from build123d import *


with BuildPart() as part:
    # Sketch1 → Base-Revolve (revolve)
    with BuildSketch(Plane.XY):
        with BuildLine():
            Line((163, 32.5), (0, 32.5))
            Line((0, 32.5), (-162.6, 32.5))
            ThreePointArc((-162.6, 32.5), (-162.882842712, 32.382842712), (-163, 32.1))
            Line((-163, 32.1), (-163, 28.4))
            ThreePointArc((-163, 28.4), (-163.117157288, 28.117157288), (-163.4, 28))
            Line((-163.4, 28), (-164, 28))
            Line((-164, 28), (-164, 25.230940108))
            ThreePointArc((-164, 25.230940108), (-164.053589838, 25.030940108), (-164.2, 24.884529946))
            Line((-164.2, 24.884529946), (-167.8, 22.806068977))
            ThreePointArc((-167.8, 22.806068977), (-167.946410162, 22.659658816), (-168, 22.459658816))
            Line((-168, 22.459658816), (-168, 5.1))
            Line((-168, 5.1), (-148, 5.1))
            Line((-148, 5.1), (-145.055513627, 0))
            Line((-145.055513627, 0), (147.055513627, 0))
            Line((147.055513627, 0), (150, 5.1))
            Line((150, 5.1), (170, 5.1))
            Line((170, 5.1), (170, 30.971851993))
            ThreePointArc((170, 30.971851993), (169.819152044, 31.54542843), (169.342020143, 31.911544614))
            Line((169.342020143, 31.911544614), (168.165693163, 32.339692621))
            ThreePointArc((168.165693163, 32.339692621), (167.997321197, 32.384807753), (167.823673019, 32.4))
            Line((167.823673019, 32.4), (165.65, 32.4))
            Line((165.65, 32.4), (165.65, 31))
            Line((165.65, 31), (163, 31))
            Line((163, 31), (163, 32.5))
        make_face()
    revolve(axis=Axis((-168, 0, 0), (1, 0, 0)))


solid = part.part
Geometry check sheet. Reference: the model listing, model coordinates, mm. A direction names the side the tool comes from. Round coordinates to 2 decimals unless told otherwise and drop trailing zeros. Write each loop counter-clockwise with the first axis right and the second up, starting at its lowest first coordinate (ties: lowest second). Pieces come first, ordered by that corner, then holes.
Item 1: Material ranges on line 1 along Z through (x, y) = (165.5, 0); line 2 along Z through (x, y) = (155, 0); line 3 along X through (y, z) = (-28, 14), recorded low to high.
Determined:
line 1: z = -31 to -5.1, 5.1 to 31
line 2: z = -32.5 to -5.1, 5.1 to 32.5
line 3: x = -163 to 163, 165.65 to 169.94
Item 2: Section check A-A (x = -39.5). Record the boundary of the cut face in (y, z).
Determined:
outline: circle Ø65 at (0, 0)
Item 3: Go/stop test with flat-tipped pins: pin 1 Ø1.5 at (x, y) = (127, 6.5) entering from -Z; pin 2 Ø5 at (y, z) = (20, -25) entering from -X; pin 3 Ø8 at (y, z) = (0, 0) entering from -X. Record where each tip stops, or that it passes through.
Determined:
pin 1: stops at z = -31.99
pin 2: stops at x = -163
pin 3: stops at x = -147.36
Item 4: Mould release check, pull along Y, two halves, no side actions. Record for faces 1 (the face through (-168, -0.3, 5.3)), 2 (the face through (-2.08, 31, 9.76)), 3 (the face through (147.57, 0.41, -0.79)): +Y half, -Y half, draft (parallel to the pull), parting line (faces both ways), or undercut.
Determined:
face 1: draft
face 2: parting line
face 3: undercut
Item 5: Access from +Z, -Z, +X, -X, +Y, -Y to the whole of each face (thin tool, end or side, straight path). Record for faces 4 (the face through (-157.9, 2.4, -4.5)), 5 (the face through (165.65, 12, -29)), 6 (the face through (160.1, 2.4, -4.5)).
Determined:
face 4: -X
face 5: none
face 6: +X
